```python
from build123d import *

# Parameters (mm, degrees)
SKETCH1_W           = 44.45
SKETCH1_H           = 19.05
BOSS_EXTRUDE1_DEPTH = 88.9
SKETCH3_R           = 7.9375
CUT_EXTRUDE1_DEPTH  = 20.05


with BuildPart() as part:
    # Sketch1 → Boss-Extrude1 (new body)
    with BuildSketch(Plane.XY):
        Rectangle(SKETCH1_W, SKETCH1_H)
    extrude(amount=-BOSS_EXTRUDE1_DEPTH)

    # Sketch3 → Cut-Extrude1 (cut, through all)
    with BuildSketch(Plane(origin=(0, 9.525, 0), x_dir=(1, 0, 0), z_dir=(0, 1, 0))):
        with Locations((12.7, 44.45)):
            Circle(SKETCH3_R)
    extrude(amount=-CUT_EXTRUDE1_DEPTH, mode=Mode.SUBTRACT)


solid = part.part
```
Can you work these out from the model? Positions are in its coordinate system, mm. Round coordinates to 2 decimals unless told otherwise and drop trailing zeros. Loops run counter-clockwise (first coordinate to the right, second up) from the corner with the lowest first, then second, coordinate; pieces in that order, holes last.
Item 1: Suppose I cut it at A-A, the plane x = 12.7. Write out the boundary of the cut face in (y, z) (1 decimal).
Item 2: Suppose I cut it at B-B, the plane z = -44.45. Write out the boundary of the cut face in (x, y) (1 decimal).
Item 3: If we mould it in two halves opening along X, with no side actions, what happens to faces 1 (the flat face through (-22.225, 0, -44)), 2 (the cylindrical face through (10.98, 0.13, -36.7)), 3 (the flat face through (0, 9.525, -44)), 4 (the flat face through (22.225, 0, -44))? For each: +X half, -X half, draft (parallel to the pull), parting line (faces both ways), or undercut.
Item 4: Please list where these lines run through material, in increasing order: L1, parallel to Z at x = 12.7, y = -2.25; L2, parallel to X at y = 5, z = -44.45 (1 decimal); L3, parallel to Z at x = 6, y = 8.75.
Reported:
1. outline: (-9.5, -88.9) - (9.5, -88.9) - (9.5, -52.4) - (-9.5, -52.4) - close; (-9.5, -36.5) - (9.5, -36.5) - (9.5, 0) - (-9.5, 0) - close
2. outline: (-22.2, -9.5) - (4.8, -9.5) - (4.8, 9.5) - (-22.2, 9.5) - close; (20.6, -9.5) - (22.2, -9.5) - (22.2, 9.5) - (20.6, 9.5) - close
3. face 1: -X half
3. face 2: undercut
3. face 3: draft
3. face 4: +X half
4. L1: z = -88.9 to -52.39, -36.51 to 0
4. L2: x = -22.2 to 4.8, 20.6 to 22.2
4. L3: z = -88.9 to -48.71, -40.19 to 0
